Check sheet for the drawn part. Datum: minimum x, y, z corner. Units: mm. Round coordinates to 2 decimals unless told otherwise and drop trailing zeros. Loops run counter-clockwise (first coordinate to the right, second up) from the corner with the lowest first, then second, coordinate; pieces in that order, holes last. Notation, with made-up numbers: (-14.75, 71.5) -> (20.25, 71.5) arc R13 cw to (20.25, 90.5) -> close; hole circle Ø4 at (-27.5, -9). An arc over 180 degrees is marked (long way). Return JSON: item names as keys, results as strings.
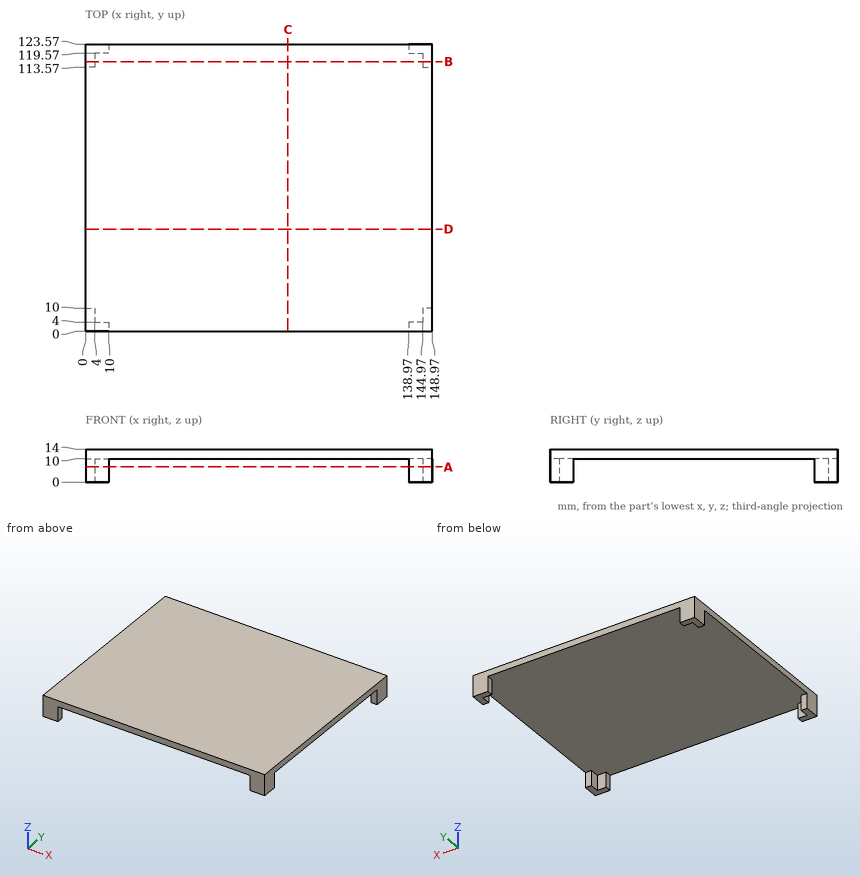
Q1. Section check A-A (z = 6.5). Record the boundary of the cut face in (x, y), then the cut area to 3 significant figures.
Results list:
{"outline": "(0, 0) -> (10, 0) -> (10, 4) -> (4, 4) -> (4, 10) -> (0, 10) -> close; (0, 113.57) -> (4, 113.57) -> (4, 119.57) -> (10, 119.57) -> (10, 123.57) -> (0, 123.57) -> close; (138.97, 0) -> (148.97, 0) -> (148.97, 10) -> (144.97, 10) -> (144.97, 4) -> (138.97, 4) -> close; (138.97, 119.57) -> (144.97, 119.57) -> (144.97, 113.57) -> (148.97, 113.57) -> (148.97, 123.57) -> (138.97, 123.57) -> close", "area": "256 mm^2"}
Q2. Material ranges on line 1 (X direction, y = 118, z = 1); line 2 (Z direction, x = 90, y = 118), recorded low to high.
Results list:
{"line 1": "0 to 4, 144.97 to 148.97", "line 2": "10 to 14"}
Q3. Go/stop test with flat-tipped pins: pin 1 (1 mm diameter, centred on x = 17.5, y = 51.5, fed in from -Z); pin 2 (1.5 mm diameter, centred on x = 56, z = 8.5, fed in from +Y). Record where each tip stops, or that it passes through.
Results list:
{"pin 1": "z = 10", "pin 2": "through"}
Q4. Section check D-D (y = 44). Record the boundary of the cut face in (x, z), then the cut area to 3 significant figures.
Results list:
{"outline": "(0, 10) -> (148.97, 10) -> (148.97, 14) -> (0, 14) -> close", "area": "596 mm^2"}
Q5. Section check B-B (y = 116). Record the boundary of the cut face in (x, z).
Results list:
{"outline": "(0, 0) -> (4, 0) -> (4, 10) -> (144.97, 10) -> (144.97, 0) -> (148.97, 0) -> (148.97, 14) -> (0, 14) -> close"}
Q6. Section check C-C (x = 87). Record the boundary of the cut face in (y, z).
Results list:
{"outline": "(0, 10) -> (123.57, 10) -> (123.57, 14) -> (0, 14) -> close"}
